Here's how the part is built. I have some questions about the finished solid (model axes, mm). A direction names the side the tool comes from. Round coordinates to 2 decimals unless told otherwise and drop trailing zeros. Order: outer loops, then holes, each group sorted by start corner. A loop starts at its lowest first (then second) coordinate and runs counter-clockwise, first axis right, second up. Notation, with made-up numbers: (-5.75, 83.5) - (48.25, 83.5) arc R29 cw to (48.25, 114.5) - close; hole circle Ø5 at (65, -2.75). An arc over 180 degrees is marked (long way). Answer as a JSON object with one key per item and string values.
```python
from build123d import *

# Parameters (mm, degrees)
SALIENTE_EXTRUIR1_DEPTH = 4
CROQUIS2_W              = 22
CROQUIS2_H              = 42
CORTAR_EXTRUIR1_DEPTH   = 4


with BuildPart() as part:
    # Croquis1 → Saliente-Extruir1 (new body)
    with BuildSketch(Plane.XY):
        with BuildLine():
            Line((0, 0), (10, 0))
            Line((10, 0), (10, 4))
            Line((10, 4), (25, 4))
            Line((25, 4), (25, 0))
            Line((25, 0), (35, 0))
            Line((35, 0), (35, 4))
            Line((35, 4), (50, 4))
            Line((50, 4), (50, 0))
            Line((50, 0), (60, 0))
            Line((60, 0), (60, 4))
            Line((60, 4), (75, 4))
            Line((75, 4), (75, 0))
            Line((75, 0), (85, 0))
            Line((85, 0), (85, 40))
            ThreePointArc((85, 40), (42.5, 82.5), (0, 40))
            Line((0, 40), (0, 0))
        make_face()
    extrude(amount=SALIENTE_EXTRUIR1_DEPTH)

    # Croquis2 → Cortar-Extruir1 (cut)
    with BuildSketch(Plane.XY.offset(4)):
        with Locations((42.5, 48)):
            Rectangle(CROQUIS2_W, CROQUIS2_H)
    extrude(amount=-CORTAR_EXTRUIR1_DEPTH, mode=Mode.SUBTRACT)


solid = part.part
```
1. For P1, Ø2, axis at x = 39, z = 2, coming from the +Y side; P2, Ø1.2, axis at x = 69.5, z = 1.5, coming from the -Y side; P3, Ø2, axis at y = 2, z = 1.5, coming from the -X side; P4, Ø1.5, axis at y = 67.5, z = 3, coming from the -X side, each with a flat end and sliding along its axis, tell me the tip position at first contact or that it passes through.
Responses:
{"P1": "y = 82.43", "P2": "y = 4", "P3": "x = 0", "P4": "x = 9.47"}
2. Imagine slicing it at A-A (x = 42.5). List the corners of the cut face in (y, z) for me, plus the area to 3 significant figures.
Responses:
{"outline": "(4, 0) - (27, 0) - (27, 4) - (4, 4) - close; (69, 0) - (82.5, 0) - (82.5, 4) - (69, 4) - close", "area": "146 mm2"}
3. If I drill on L1, parallel to X at y = 36.5, z = 1.45; L2, parallel to Y at x = 43, z = 2; L3, parallel to X at y = 47.5, z = 3.4, over which ranges is the centre line in solid material (lowest first)? Write a range as [from, to].
Responses:
{"L1": "[0, 31.5], [53.5, 85]", "L2": "[4, 27], [69, 82.5]", "L3": "[0.67, 31.5], [53.5, 84.33]"}
4. Imagine slicing it at B-B (y = 28). List the corners of the cut face in (x, z) for me, plus the area to 3 significant figures.
Responses:
{"outline": "(0, 0) - (31.5, 0) - (31.5, 4) - (0, 4) - close; (53.5, 0) - (85, 0) - (85, 4) - (53.5, 4) - close", "area": "252 mm2"}
5. For faces 5 (the face through (25, 2, 2)), 6 (the face through (42, 69, 2)), 7 (the face through (43.43, 82.49, 1.97)), which set-ups out of +Z, -Z, +X, -X, +Y, -Y let a thin tool reach every point of the face, with its end or its side?
Responses:
{"face 5": "+Z, -Z, -Y", "face 6": "+Z, -Z", "face 7": "+Z, -Z, +Y"}
6. Thinking about a two-plate mould opening in Y: for faces 1 (the face through (53.5, 48, 2)), 2 (the face through (42, 27, 2)), 3 (the face through (50, 2, 2)), 4 (the face through (42, 4, 2)), which applies, pulls with the +Y half, pulls with the -Y half, needs draft (parallel to the pull), parting line crosses it, or undercut?
Responses:
{"face 1": "undercut", "face 2": "undercut", "face 3": "needs draft", "face 4": "pulls with the -Y half"}
7. Imagine slicing it at D-D (x = 13). List the corners of the cut face in (y, z) for me, plus the area to 3 significant figures.
Responses:
{"outline": "(4, 0) - (70.59, 0) - (70.59, 4) - (4, 4) - close", "area": "266 mm2"}
8. Imagine slicing it at C-C (z = 1.6). List the corners of the cut face in (x, y) for me, plus the area to 3 significant figures.
Responses:
{"outline": "(0, 0) - (10, 0) - (10, 4) - (25, 4) - (25, 0) - (35, 0) - (35, 4) - (50, 4) - (50, 0) - (60, 0) - (60, 4) - (75, 4) - (75, 0) - (85, 0) - (85, 40) arc R42.5 ccw to (0, 40) - close; hole (31.5, 27) - (53.5, 27) - (53.5, 69) - (31.5, 69) - close", "area": "5,130 mm2"}
